Part print with two shaded views. Sizes in mm from the minimum x, y, z corner. A direction names the side the tool comes from. Coordinates: 2 decimals unless noted, no trailing zeros. Loops run counter-clockwise (first coordinate to the right, second up) from the corner with the lowest first, then second, coordinate; pieces in that order, holes last.
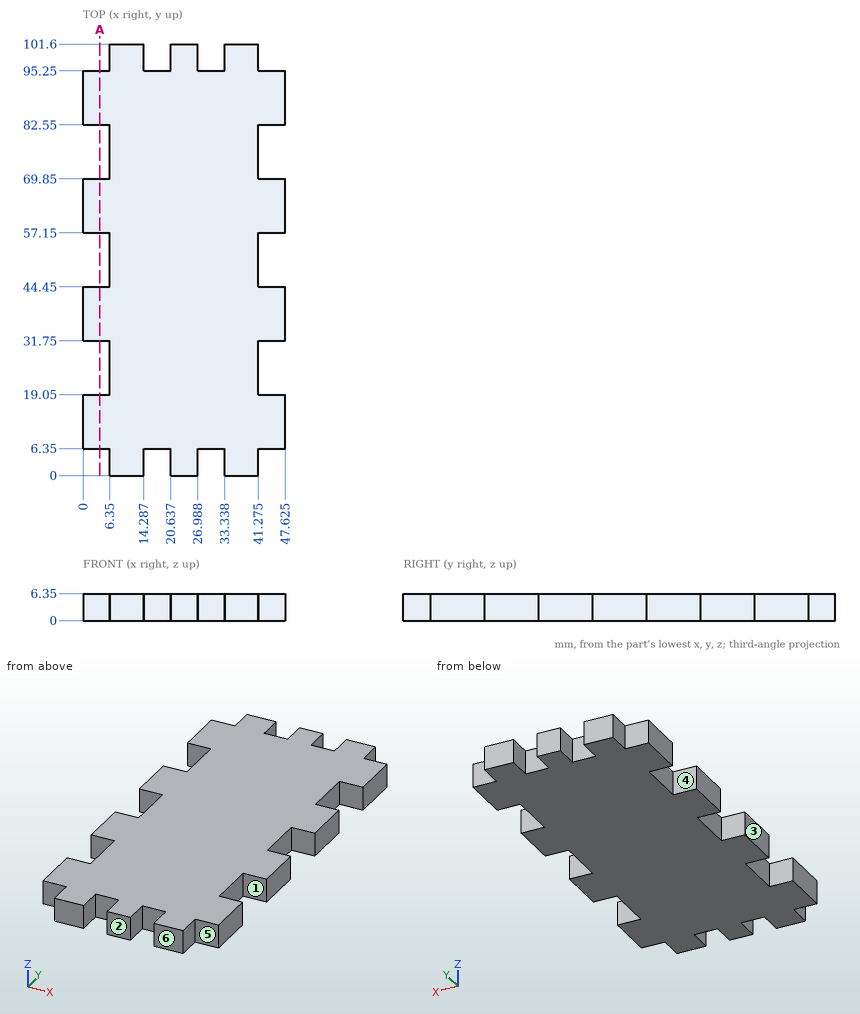
Q1. Flat gauge pins, fed straight in: P1, Ø3, axis at x = 45, z = 1.5, coming from the -Y side; P2, Ø3, axis at x = 2.5, z = 2, coming from the +Y side; P3, Ø3, axis at y = 4.5, z = 1.5, coming from the +X side (1 decimal). Where does each tip first touch, or does it go through?
Answers:
P1: stops at y = 6.35
P2: stops at y = 95.25
P3: stops at x = 41.3
Q2. Which spindle directions (+Z, -Z, +X, -X, +Y, -Y) get a long thin tool onto all of the face, cutting with end or side? Do the marked faces 4, 5 and 6. Say none if no direction does.
Answers:
face 4: +Z, -Z, -X
face 5: +Z, -Z, +X, -Y
face 6: +Z, -Z, +X, -X, -Y
Q3. Drill centre lines: line 1 (Y direction, x = 43, z = 3.5); line 2 (Y direction, x = 33, z = 1.5). Where is each one in solid material? Low to high.
Answers:
line 1: y = 6.35 to 19.05, 31.75 to 44.45, 57.15 to 69.85, 82.55 to 95.25
line 2: y = 6.35 to 95.25
Q4. Mould opens along Y. For the marked faces 1, 2 and 3 say: +Y half, -Y half, draft (parallel to the pull), parting line (faces both ways), or undercut.
Answers:
face 1: undercut
face 2: -Y half
face 3: draft
Q5. Slice it at A-A (x = 4). List the corners of the cut face in (y, z).
Answers:
outline: (6.35, 0) - (19.05, 0) - (19.05, 6.35) - (6.35, 6.35) - close; (31.75, 0) - (44.45, 0) - (44.45, 6.35) - (31.75, 6.35) - close; (57.15, 0) - (69.85, 0) - (69.85, 6.35) - (57.15, 6.35) - close; (82.55, 0) - (95.25, 0) - (95.25, 6.35) - (82.55, 6.35) - close
